from build123d import *

# Parameters (mm, degrees)
M5_GEWINDEBOHRUNG2_D     = 4.2
M5_GEWINDEBOHRUNG2_DEPTH = 12
M5_GEWINDEBOHRUNG2_TIP   = 1.2618073
VERRUNDUNG1_R            = 2


with BuildPart() as part:
    # Skizze1 → Rotation1 (revolve)
    with BuildSketch(Plane.XY):
        Polygon((0, 0), (0, 7.5), (0.5, 7.5), (0.5, 19), (25.5, 19), (25.5, 7.5), (26, 7.5), (26, 0), align=None)
    revolve(axis=Axis((0, 0, 0), (1, 0, 0)))

    # Skizze2 → M5 Gewindebohrung1 (revolve, cut)
    with BuildSketch(Plane(origin=(26, 0, 0), x_dir=(0, 0, -1), z_dir=(0, 1, 0))):
        Polygon((0, 0), (0, 13.2618073), (2.1, 12), (2.1, 0), align=None)
    revolve(axis=Axis((32.35, 0, 0), (-1, 0, 0)), mode=Mode.SUBTRACT)

    # M5 Gewindebohrung2
    with Locations(Plane.ZY):
        with Locations((0, 0)):
            Hole(M5_GEWINDEBOHRUNG2_D / 2, depth=M5_GEWINDEBOHRUNG2_DEPTH)
            with Locations((0, 0, -(M5_GEWINDEBOHRUNG2_DEPTH + M5_GEWINDEBOHRUNG2_TIP / 2))):  # 118° drill point
                Cone(0, M5_GEWINDEBOHRUNG2_D / 2, M5_GEWINDEBOHRUNG2_TIP, mode=Mode.SUBTRACT)

    # Verrundung1
    verrundung1_edges = [part.edges().sort_by_distance(p)[0] for p in [
        (0.5, -19, 0),
        (25.5, -19, 0),
    ]]
    fillet(verrundung1_edges, radius=VERRUNDUNG1_R)


solid = part.part
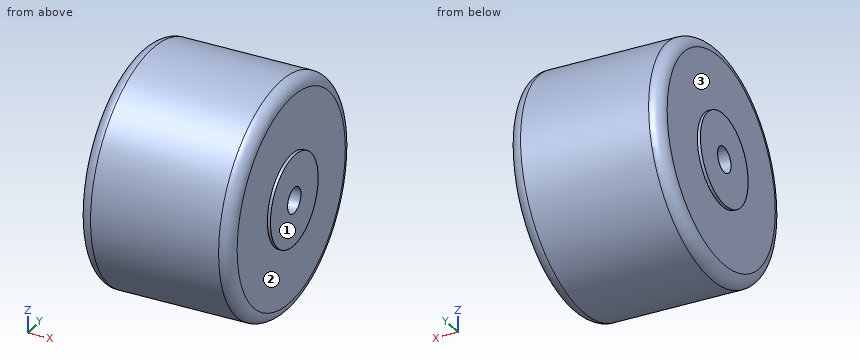
Part model, mm, in its own coordinate system. Face numbers are marked on the shaded views. A direction names the side the tool comes from. Round coordinates to 2 decimals unless told otherwise and drop trailing zeros. Loops run counter-clockwise (first coordinate to the right, second up) from the corner with the lowest first, then second, coordinate; pieces in that order, holes last. Notation, with made-up numbers: (-7.75, -24) - (40.25, -24) arc R12 cw to (40.25, -7) - close; hole circle Ø2 at (2, -30.75). An arc over 180 degrees is marked (long way). Answer as a JSON object with one key per item and string values.
Item 1: Band-saw the part on A-A on y = 0. List the corners of the cut face in (x, z).
Output:
{"outline": "(0, -7.5) - (0.5, -7.5) - (0.5, -17) arc R2 ccw to (2.5, -19) - (23.5, -19) arc R2 ccw to (25.5, -17) - (25.5, -7.5) - (26, -7.5) - (26, -2.1) - (14, -2.1) - (13, -0.44) - (12, -2.1) - (0, -2.1) - close; (0, 2.1) - (12, 2.1) - (13, 0.44) - (14, 2.1) - (26, 2.1) - (26, 7.5) - (25.5, 7.5) - (25.5, 17) arc R2 ccw to (23.5, 19) - (2.5, 19) arc R2 ccw to (0.5, 17) - (0.5, 7.5) - (0, 7.5) - close"}
Item 2: Tool access for the marked faces 1, 2 and 3: list every direction of +Z, -Z, +X, -X, +Y, -Y with a clear straight run to the whole face (end or side of a thin tool).
Output:
{"face 1": "+Z, -Z, +X, +Y, -Y", "face 2": "+X", "face 3": "-X"}
Item 3: Pin check, flat tips, straight feed: pin 1 (6 mm diameter, centred on x = 14.5, z = 7.5, fed in from -Y); pin 2 (6 mm diameter, centred on x = 19.5, y = -4.5, fed in from -Z); pin 3 (4 mm diameter, centred on y = -14.5, z = 10.5, fed in from +X). Stop position of each tip, or through.
Output:
{"pin 1": "y = -18.46", "pin 2": "z = -18.94", "pin 3": "x = 25.5"}
Item 4: Wall check: L1, parallel to Z at x = 17.75, y = 0; L2, parallel to X at y = 13, z = 1.5; L3, parallel to Y at x = 20.5, z = -8.5. Give the ranges that are in metal, low to high.
Output:
{"L1": "-19 to -2.1, 2.1 to 19", "L2": "0.5 to 25.5", "L3": "-16.99 to 16.99"}
Item 5: Band-saw the part on B-B on x = 10. List the corners of the cut face in (y, z), plus the area to 3 significant figures.
Output:
{"outline": "circle Ø38 at (0, 0); hole circle Ø4.2 at (0, 0)", "area": "1,120 mm2"}
